Solid Edge part; units mm, degrees
sketch "Sketch1" plane through (0, 0, 0) normal (0, 0, 1) x (1, 0, 0)
  line L0 (105.1974, 149.4572) -> (268.1974, 149.4572)
  line L1 (268.1974, 149.4572) -> (268.1974, 19.4572)
  line L2 (268.1974, 19.4572) -> (105.1974, 19.4572)
  line L3 (105.1974, 19.4572) -> (105.1974, 149.4572)
  dimension "D1" = 105.1974
  dimension "D2" = 268.1974
extrude "Protrusion1" add sketch "Sketch1" along normal blind 27
sketch "Sketch2" plane through (170.1974, 84.4572, 27) normal (0, 0, 1) x (1, 0, 0)
  line L0 (-62, 62) -> (-62, -62)
  line L1 (-62, -62) -> (95, -62)
  line L2 (95, -62) -> (95, 62.14)
  line L3 (-62, 62) -> (95, 62.14)
  dimension "D1" = 62
  dimension "D2" = 95
extrude "ExtrudedCutout_1" cut sketch "Sketch2" against normal blind 23
sketch "Sketch3" plane through (170.1974, 84.5136, 4) normal (0, 0, 1) x (1, 0, 0)
  circle A0 centre (-57, -0.0564) radius 2
  circle A1 centre (-48, -0.0564) radius 2
extrude "Cutout1" cut sketch "Sketch3" against normal through all
sketch "Sketch4" plane through (186.6974, 84.4572, 0) normal (0, 0, -1) x (1, 0, 0)
  circle A0 centre (17.5, 0) radius 62
extrude "Cutout2" cut sketch "Sketch4" against normal through all
sketch "Sketch5" plane through (268.1974, 84.4572, 13.5) normal (1, 0, 0) x (0, 0, 1)
  line L0 (13.5, 0) -> (13.5, 5)
  line L1 (13.5, 5) -> (3.5, 5)
  line L2 (3.5, -5) -> (3.5, 5)
  line L3 (13.5, -5) -> (3.5, -5)
  line L4 (13.5, 0) -> (13.5, -5)
  dimension "D1" = 13.5
  dimension "D2" = 13.5
  dimension "D3" = 13.5
  dimension "D4" = 13.5
extrude "ExtrudedProtrusion_7" add sketch "Sketch5" along normal blind 10
sketch "Sketch6" plane through (273.1974, 84.4572, 17) normal (0, 0, -1) x (1, 0, 0)
  circle A0 centre (0, 0) radius 2
extrude "Cutout3" cut sketch "Sketch6" against normal through all
sketch "Sketch7" plane through (191.6974, 84.4572, 27) normal (0, 0, 1) x (1, 0, 0)
  line L0 (-122.0031, 91.8624) -> (-122.0031, -126.2255)
  line L1 (-122.0031, -126.2255) -> (122.899, -118.4792)
  line L2 (122.899, -118.4792) -> (110.9816, 91.8624)
  line L3 (110.9816, 91.8624) -> (-122.0031, 91.8624)
extrude "ExtrudedCutout_10" cut sketch "Sketch7" against normal blind 1
Input: part model. Units: mm. Frame: model coordinates. A direction names the side the tool comes from. Coordinates: 2 decimals unless noted, no trailing zeros. Loops run counter-clockwise (first coordinate to the right, second up) from the corner with the lowest first, then second, coordinate; pieces in that order, holes last. Notation, with made-up numbers: M -26,51.25 L -7,51.25 A14 ccw -7,59.25 Z; hole C 49.25,46.5 d4. An arc over 180 degrees is marked long. Use a Markdown table: item, result. Add a question column.
1) Draft query along X for faces 1 (the flat face through (108.197, 85, 15)), 2 (the flat face through (105.197, 84, 13)), 3 (the flat face through (273, 82, 17)). Return one class per face: +X half, -X half, draft (parallel to the pull), parting line (faces both ways), or undercut.
2) Section D-D, the plane z = 24. Return the cut outline in (x, y).
3) Section A-A, the plane z = 9.25. Return the cut outline in (x, y).
4) Set-up query: faces 4 (the flat face through (250, 37, 4)), 5 (the flat face through (273, 89.457, 22)), 6 (the flat face through (273, 79.457, 22)). Return all of +Z, -Z, +X, -X, +Y, -Y with unobstructed straight access to the full face (end or side cutting, diameter ignored); none if empty.
5) Section C-C, the plane x = 183.5. Return the cut outline in (y, z), plus the area to 3 significant figures.
6) Section B-B, the plane y = 55. Return the cut outline in (x, z), plus the area to 3 significant figures.
7) Pin query (flat end, axial travel): P1, Ø8, axis at x = 247.5, y = 132, coming from the -Z side; P2, Ø2.5, axis at x = 271, z = 22, coming from the +Y side; P3, Ø2.5, axis at x = 272, z = 23.5, coming from the -Y side; P4, Ø4.5, axis at x = 273.2, y = 84.46, coming from the -Z side. Return the tip coordinate at first contact, or that it passes through.
8) Line query: L1, parallel to X at y = 137.5, z = 12; L2, parallel to Y at x = 134, z = 17.25; L3, parallel to Y at x = 218, z = 13.75. Output: solid intervals per line, ascending. Write a range as from..to.
Answer below:
| question | item | result |
|---|---|---|
| 1 | face 1 | undercut |
| 1 | face 2 | -X half |
| 1 | face 3 | draft |
| 2 | outline | M 105.2,19.46 L 268.2,19.46 L 268.2,79.46 L 278.2,79.46 L 278.2,89.46 L 268.2,89.46 L 268.2,149.46 L 105.2,149.46 Z; hole M 108.2,22.46 L 265.2,22.46 L 265.2,73.37 A62 ccw 265.2,95.55 L 265.2,146.6 L 108.2,146.46 Z; hole C 273.2,84.46 d4 |
| 3 | outline | M 105.2,19.46 L 268.2,19.46 L 268.2,149.46 L 105.2,149.46 Z; hole M 108.2,22.46 L 265.2,22.46 L 265.2,73.37 A62 ccw 265.2,95.55 L 265.2,146.6 L 108.2,146.46 Z |
| 4 | face 4 | +Z |
| 4 | face 5 | +Z, -Z, +X, +Y |
| 4 | face 6 | +Z, -Z, +X, -Y |
| 5 | outline | M 19.46,0 L 26.01,0 L 26.01,4 L 22.46,4 L 22.46,26 L 19.46,26 Z; M 142.9,0 L 149.46,0 L 149.46,26 L 146.52,26 L 146.52,4 L 142.9,4 Z |
| 5 | area | 183 mm2 |
| 6 | outline | M 105.2,0 L 149.64,0 L 149.64,4 L 108.2,4 L 108.2,26 L 105.2,26 Z; M 258.75,0 L 268.2,0 L 268.2,26 L 265.2,26 L 265.2,4 L 258.75,4 Z |
| 6 | area | 348 mm2 |
| 7 | P1 | z = 0 |
| 7 | P2 | y = 89.46 |
| 7 | P3 | y = 79.46 |
| 7 | P4 | z = 17 |
| 8 | L1 | 105.2..108.2, 265.2..268.2 |
| 8 | L2 | 19.46..22.46, 146.48..149.46 |
| 8 | L3 | 19.46..22.46, 146.56..149.46 |
